Design review of the part shown in the three views and the two pictorial views. Dimensions are in mm from the part's minimum x, y and z. A direction names the side the tool comes from. Give positions to 0.01 mm unless a question says otherwise; leave off trailing zeros. Loops run counter-clockwise (first coordinate to the right, second up) from the corner with the lowest first, then second, coordinate; pieces in that order, holes last. Notation, with made-up numbers: (70, -26.5) -> (97, -26.5) arc R8 cw to (97, -11.5) -> close; hole circle Ø10 at (52, 79). An arc over 180 degrees is marked (long way). Answer as CSV lines item,"result". Start each with the question number.
Item 1: Clearance check with flat-ended pins moving along their axes: P1, Ø6, axis at x = 38.5, z = 22, coming from the +Y side; P2, Ø5, axis at y = 13, z = 17.5, coming from the +X side; P3, Ø6, axis at x = 21.5, z = 34, coming from the +Y side; P4, Ø4, axis at y = 28.5, z = 23.5, coming from the +X side. State where each tip first meets the part, or that it passes through.
Item 2: Add section B-B on z = 30.5. State the section outline as (x, y) points (1 decimal), plus the area to 3 significant figures.
Item 3: Machinability: for the marked faces 1 and 2, which of the approach directions +Z, -Z, +X, -X, +Y, -Y give a long, thin tool a straight path to every point of the face, cutting with its end or side? Answer none if there is none.
Item 4: Add section D-D on x = 20. State the section outline as (y, z) points (1 decimal).
Item 5: Add section A-A on x = 29.5. State the section outline as (y, z) points, plus the area to 3 significant figures.
Item 6: The part is to be moulded in two halves that separate along X. For the marked faces 3 and 4, say which applies: +X half, -X half, draft (parallel to the pull), parting line (faces both ways), or undercut.
Item 7: For L1, parallel to Y at x = 4.5, z = 30; L2, parallel to Y at x = 27, z = 43.5; L3, parallel to X at y = 11.5, z = 43 (1 decimal), list the stretches that pass through material, from the lowest coordinate up. Write a range as from..to.
Item 8: Add section C-C on y = 26.5. State the section outline as (x, z) points (1 decimal).
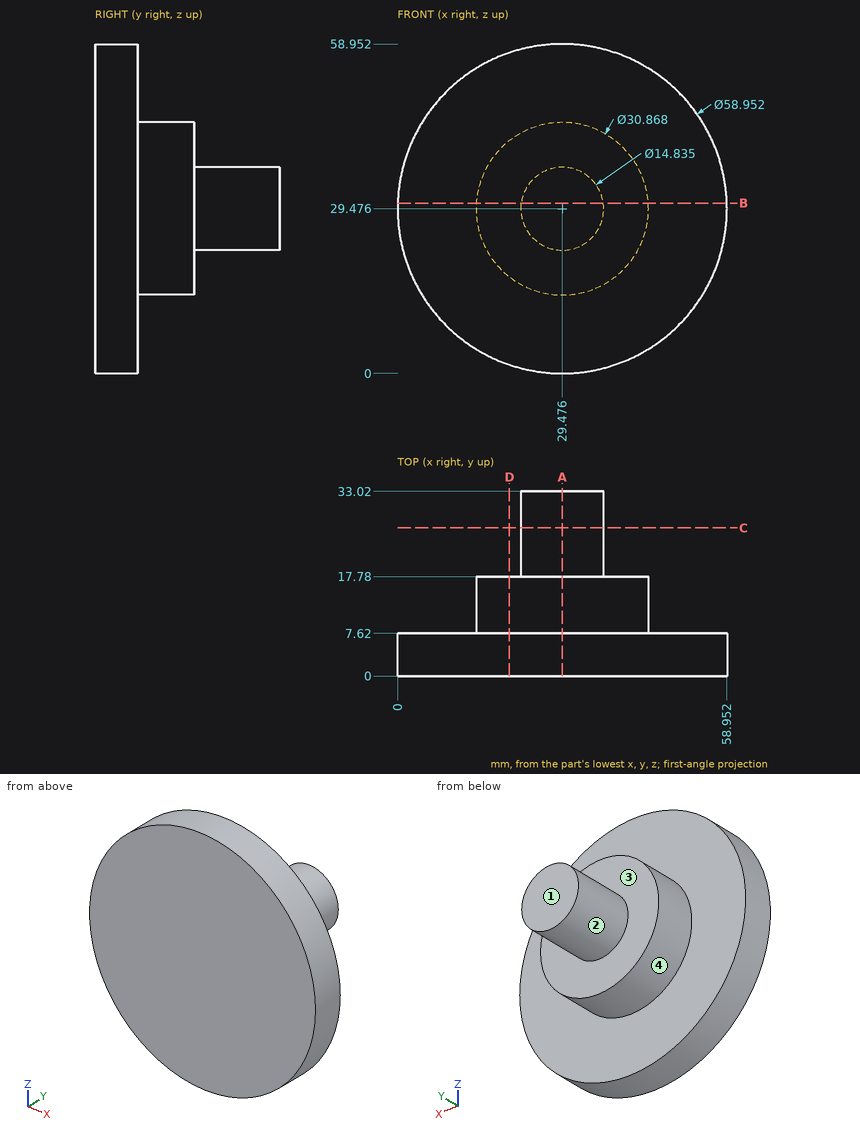
Computed values:
1,P1,"y = 17.78"
1,P2,"x = 41.66"
1,P3,"y = 33.02"
1,P4,"x = 35.74"
2,outline,"(0, 0) -> (58.9, 0) -> (58.9, 7.6) -> (44.9, 7.6) -> (44.9, 17.8) -> (36.8, 17.8) -> (36.8, 33) -> (22.1, 33) -> (22.1, 17.8) -> (14.1, 17.8) -> (14.1, 7.6) -> (0, 7.6) -> close"
2,area,"986 mm²"
3,face 1,"+Z, -Z, +X, -X, +Y"
3,face 2,"+Y"
4,outline,"(0, 1.6) -> (7.6, 1.6) -> (7.6, 17.3) -> (17.8, 17.3) -> (17.8, 41.7) -> (7.6, 41.7) -> (7.6, 57.4) -> (0, 57.4) -> close"
5,outline,"(0, 0) -> (7.62, 0) -> (7.62, 14.04) -> (17.78, 14.04) -> (17.78, 22.06) -> (33.02, 22.06) -> (33.02, 36.89) -> (17.78, 36.89) -> (17.78, 44.91) -> (7.62, 44.91) -> (7.62, 58.95) -> (0, 58.95) -> close"
5,area,"989 mm²"
6,face 3,"draft"
6,face 4,"parting line"
7,L1,"0..7.62"
7,L2,"0..17.78"
7,L3,"22..36.9"
8,outline,"circle Ø14.8 at (29.5, 29.5)"
